```python
from build123d import *

# Parameters (mm, degrees)
RESSALTO_EXTRUS_O1_DEPTH = 2
RESSALTO_EXTRUS_O2_DEPTH = 7


with BuildPart() as part:
    # Esboço1 → Ressalto-extrusão1 (new body)
    with BuildSketch(Plane(origin=(0, 0, 0), x_dir=(1, 0, 0), z_dir=(0, 1, 0))):
        with BuildLine():
            Line((-10.348817595, -24.761398547), (9.651182405, -24.761398547))
            ThreePointArc((9.651182405, -24.761398547), (16.722250217, -21.832466359), (19.651182405, -14.761398547))
            Line((19.651182405, -14.761398547), (19.651182405, 15.238601453))
            ThreePointArc((19.651182405, 15.238601453), (16.722250217, 22.309669265), (9.651182405, 25.238601453))
            Line((9.651182405, 25.238601453), (-10.348817595, 25.238601453))
            ThreePointArc((-10.348817595, 25.238601453), (-17.419885407, 22.309669265), (-20.348817595, 15.238601453))
            Line((-20.348817595, 15.238601453), (-20.348817595, -14.761398547))
            ThreePointArc((-20.348817595, -14.761398547), (-17.419885407, -21.832466359), (-10.348817595, -24.761398547))
        make_face()
    extrude(amount=RESSALTO_EXTRUS_O1_DEPTH)

    # Esboço2 → Ressalto-extrusão2 (add)
    with BuildSketch(Plane(origin=(0, 2, 0), x_dir=(1, 0, 0), z_dir=(0, 1, 0))):
        with BuildLine():
            Line((-18.748817595, 15.238601453), (-18.748817595, -14.761398547))
            ThreePointArc((-18.748817595, -14.761398547), (-16.288514557, -20.701095509), (-10.348817595, -23.161398547))
            Line((-10.348817595, -23.161398547), (9.651182405, -23.161398547))
            ThreePointArc((9.651182405, -23.161398547), (15.590879367, -20.701095509), (18.051182405, -14.761398547))
            Line((18.051182405, -14.761398547), (18.051182405, 15.238601453))
            ThreePointArc((18.051182405, 15.238601453), (15.590879367, 21.178298415), (9.651182405, 23.638601453))
            Line((9.651182405, 23.638601453), (-10.348817595, 23.638601453))
            ThreePointArc((-10.348817595, 23.638601453), (-16.288514557, 21.178298415), (-18.748817595, 15.238601453))
        make_face()
        with BuildLine():
            Line((-17.248817595, 15.238601453), (-17.248817595, -14.761398547))
            ThreePointArc((-17.248817595, -14.761398547), (-15.227854385, -19.640435337), (-10.348817595, -21.661398547))
            Line((-10.348817595, -21.661398547), (9.651182405, -21.661398547))
            ThreePointArc((9.651182405, -21.661398547), (14.530219195, -19.640435337), (16.551182405, -14.761398547))
            Line((16.551182405, -14.761398547), (16.551182405, 15.238601453))
            ThreePointArc((16.551182405, 15.238601453), (14.530219195, 20.117638244), (9.651182405, 22.138601453))
            Line((9.651182405, 22.138601453), (-10.348817595, 22.138601453))
            ThreePointArc((-10.348817595, 22.138601453), (-15.227854385, 20.117638244), (-17.248817595, 15.238601453))
        make_face(mode=Mode.SUBTRACT)
    extrude(amount=RESSALTO_EXTRUS_O2_DEPTH)


solid = part.part
```
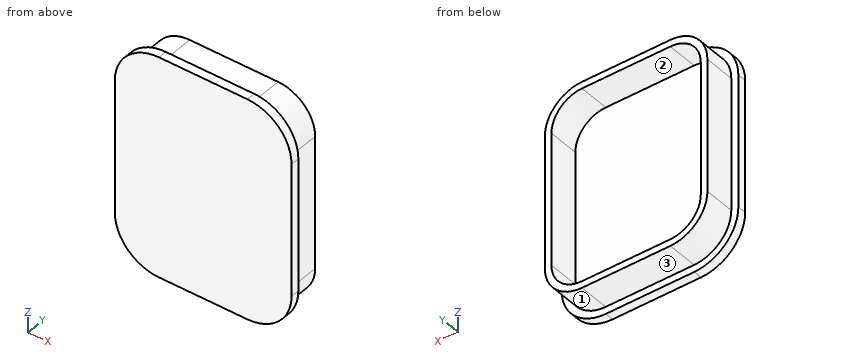
Geometry check sheet. Reference: the model listing, model coordinates, mm. Face numbers are marked on the shaded views. A direction names the side the tool comes from. Coordinates: 2 decimals unless noted, no trailing zeros. Loops run counter-clockwise (first coordinate to the right, second up) from the corner with the lowest first, then second, coordinate; pieces in that order, holes last. Notation, with made-up numbers: (47, 87.5) -> (103, 87.5) arc R19 ccw to (103, 116.5) -> close; hole circle Ø6 at (84, 57). An arc over 180 degrees is marked (long way). Put each result on its own line as item: value.
1) Tool access check on the marked faces 1, 2 and 3. Record the directions out of +Z, -Z, +X, -X, +Y, -Y that give a thin tool (end or side, any length) a straight path to the whole face; none if there is none.
Result set:
face 1: -Z, +X, +Y
face 2: +Y
face 3: -Z, +X, -X, +Y
2) Cross-section at A-A on y = 7.25. Record the boundary of the cut face in (x, z).
Result set:
outline: (-18.75, -15.24) arc R8.4 ccw to (-10.35, -23.64) -> (9.65, -23.64) arc R8.4 ccw to (18.05, -15.24) -> (18.05, 14.76) arc R8.4 ccw to (9.65, 23.16) -> (-10.35, 23.16) arc R8.4 ccw to (-18.75, 14.76) -> close; hole (-17.25, -15.24) arc R6.9 ccw to (-10.35, -22.14) -> (9.65, -22.14) arc R6.9 ccw to (16.55, -15.24) -> (16.55, 14.76) arc R6.9 ccw to (9.65, 21.66) -> (-10.35, 21.66) arc R6.9 ccw to (-17.25, 14.76) -> close
3) Thickness scan on line 1 (X direction, y = 7.75, z = -15); line 2 (Z direction, x = 8, y = 2.75); line 3 (Y direction, x = -12, z = -4). Record the ranges inside material, lowest first.
Result set:
line 1: x = -18.75 to -17.25, 16.55 to 18.05
line 2: z = -23.64 to -22.14, 21.66 to 23.16
line 3: y = 0 to 2
4) Cross-section at C-C on x = 7.5. Record the boundary of the cut face in (y, z), plus the area to 3 significant figures.
Result set:
outline: (0, -25.24) -> (2, -25.24) -> (2, -23.64) -> (9, -23.64) -> (9, -22.14) -> (2, -22.14) -> (2, 21.66) -> (9, 21.66) -> (9, 23.16) -> (2, 23.16) -> (2, 24.76) -> (0, 24.76) -> close
area: 121 mm^2
5) Gauge pin test, flat ends, axial feed: pin 1 Ø3.5 at (y, z) = (6, -5.5) entering from +X; pin 2 Ø8 at (x, z) = (8, 1.5) entering from +Y; pin 3 Ø2 at (x, y) = (-0.5, 5) entering from -Z. Record the tip position at first contact, or that the pin passes through.
Result set:
pin 1: stops at x = 18.05
pin 2: stops at y = 2
pin 3: stops at z = -23.64
6) Cross-section at B-B on z = -3. Record the boundary of the cut face in (x, y).
Result set:
outline: (-20.35, 0) -> (19.65, 0) -> (19.65, 2) -> (18.05, 2) -> (18.05, 9) -> (16.55, 9) -> (16.55, 2) -> (-17.25, 2) -> (-17.25, 9) -> (-18.75, 9) -> (-18.75, 2) -> (-20.35, 2) -> close
